Here's the drawing with two shaded views (mm, measured from the low corner). I have some questions. A direction names the side the tool comes from. Give positions to 0.01 mm unless a question says otherwise; leave off trailing zeros. Loops run counter-clockwise (first coordinate to the right, second up) from the corner with the lowest first, then second, coordinate; pieces in that order, holes last. Notation, with made-up numbers: (68, 56.25) - (72, 56.25) arc R25 ccw to (72, 75.25) - close; hole circle Ø11 at (74, 26). An arc over 180 degrees is marked (long way). Write each question's results on one line, items separated by ' | '. Start each with the question number.
1) On a 3-axis mill with a long thin cutter (end or side, diameter ignored), from which of +Z, -Z, +X, -X, +Y, -Y can I reach the whole of each face in a straight line? I mean the marked faces 1, 2, 3, 4 and 5. Say none if no direction works.
2) I'm going to push flat-ended pins straight in: pin 1 (3 mm diameter, centred on y = 4, z = 8, fed in from +X); pin 2 (1.5 mm diameter, centred on x = 18, y = 2, fed in from -Z); pin 3 (1.5 mm diameter, centred on x = 29, z = 15.5, fed in from +Y). Where does each tip first touch, or does it pass through?
3) I want a section at B-B, the plane z = 7.5. Write out the boundary of the cut face in (x, y), and give its area (3 significant figures).
4) I want a section at A-A, the plane y = 12.5. Write out the boundary of the cut face in (x, z).
5) I want a section at C-C, the plane x = 32. Write out the boundary of the cut face in (y, z), and give its area (4 significant figures).
6) I want a section at D-D, the plane y = 2.5. Write out the boundary of the cut face in (x, z).
7) If we mould it in two halves opening along Y, with no side actions, what happens to the marked faces 6, 7 and 8? For each: +Y half, -Y half, draft (parallel to the pull), parting line (faces both ways), or undercut.
8) If I drill on probe 1 along X at (y, z) = (10, 7.5); probe 2 along X at (y, z) = (12.1, 7.5); probe 3 along Z at (x, y) = (17.75, 10.35), over which ranges is the centre line in solid material (lowest first)? Write a range as [from, to].
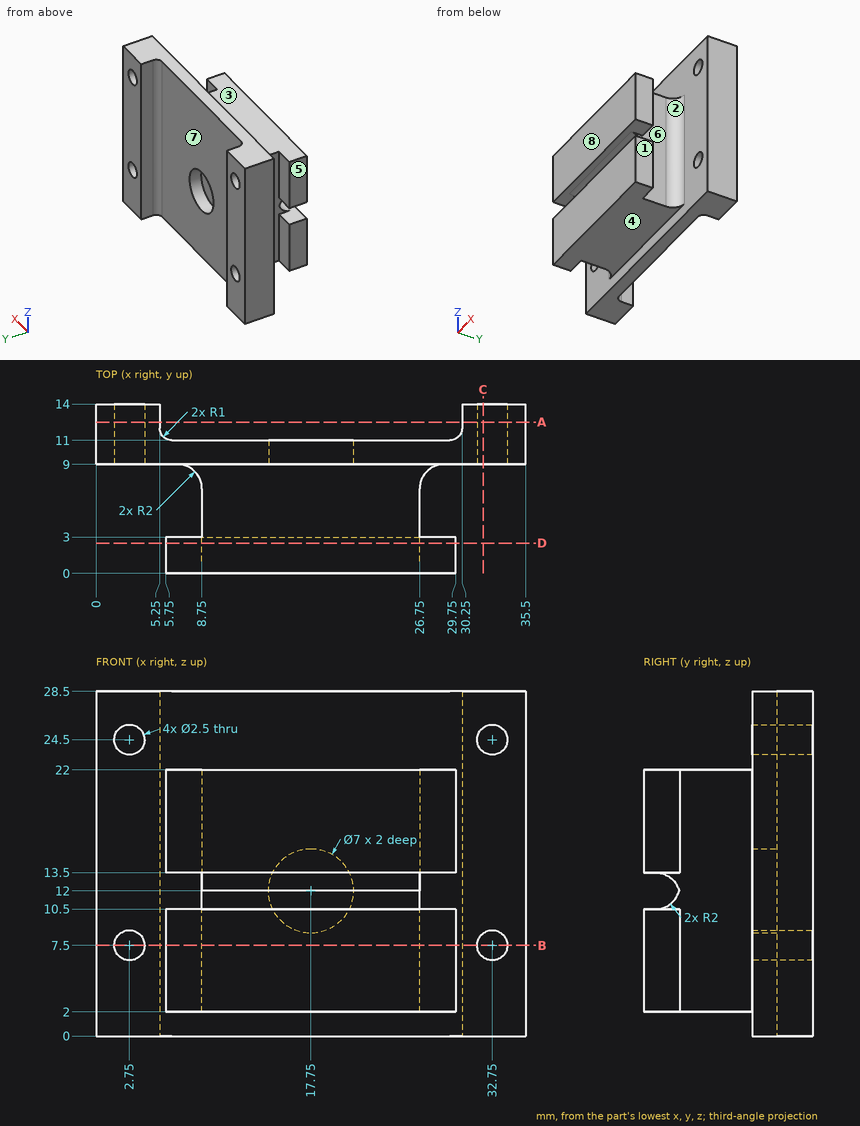
Answers:
1) face 1: +Z, -Z, +X, -Y | face 2: +Z, -Z, +X | face 3: +Z, +X, -X, -Y | face 4: -Z, +X, -X, -Y | face 5: +Z, -Z, -X, -Y
2) pin 1: stops at x = 29.75 | pin 2: stops at z = 2 | pin 3: stops at y = 11.13
3) outline: (0, 9) - (1.5, 9) - (1.5, 14) - (0, 14) - close; (4, 9) - (6.75, 9) arc R2 cw to (8.75, 7) - (8.75, 3) - (5.75, 3) - (5.75, 0) - (29.75, 0) - (29.75, 3) - (26.75, 3) - (26.75, 7) arc R2 cw to (28.75, 9) - (31.5, 9) - (31.5, 14) - (30.25, 14) - (30.25, 12) arc R1 cw to (29.25, 11) - (6.25, 11) arc R1 cw to (5.25, 12) - (5.25, 14) - (4, 14) - close; (34, 9) - (35.5, 9) - (35.5, 14) - (34, 14) - close | area: 260 mm2
4) outline: (0, 0) - (5.25, 0) - (5.25, 28.5) - (0, 28.5) - close; (30.25, 0) - (35.5, 0) - (35.5, 28.5) - (30.25, 28.5) - close; hole circle Ø2.5 at (2.75, 7.5); hole circle Ø2.5 at (2.75, 24.5); hole circle Ø2.5 at (32.75, 7.5); hole circle Ø2.5 at (32.75, 24.5)
5) outline: (9, 0) - (14, 0) - (14, 6.5) - (9, 6.5) - close; (9, 8.5) - (14, 8.5) - (14, 23.5) - (9, 23.5) - close; (9, 25.5) - (14, 25.5) - (14, 28.5) - (9, 28.5) - close | area: 122.5 mm2
6) outline: (5.75, 2) - (29.75, 2) - (29.75, 10.5) - (26.75, 10.5) - (26.75, 11.18) - (8.75, 11.18) - (8.75, 10.5) - (5.75, 10.5) - close; (5.75, 13.5) - (8.75, 13.5) - (8.75, 12.82) - (26.75, 12.82) - (26.75, 13.5) - (29.75, 13.5) - (29.75, 22) - (5.75, 22) - close
7) face 6: undercut | face 7: +Y half | face 8: -Y half
8) probe 1: x = [0, 1.5], [4, 31.5], [34, 35.5] | probe 2: x = [0, 1.5], [4, 5.25], [30.25, 31.5], [34, 35.5] | probe 3: z = [0, 8.5], [15.5, 28.5]
